Here's how the part is built. I have some questions about the finished solid (model axes, mm). A direction names the side the tool comes from. Coordinates: 2 decimals unless noted, no trailing zeros. Loops run counter-clockwise (first coordinate to the right, second up) from the corner with the lowest first, then second, coordinate; pieces in that order, holes last. Notation, with made-up numbers: M 59,63.25 L 106,63.25 A26 cw 106,89.25 Z; hole C 0.5,63 d4. An arc over 180 degrees is marked long. Use one line per item in the form item = value. Start each with the question number.
(1) Thinking about a two-plate mould opening in Z: for faces 1 (the cylindrical face through (81.769, 10.14, 82.675)), 2 (the flat face through (11.7, 9.86, 97.58)), 3 (the flat face through (-44.38, 10, -1)), 4 (the flat face through (29.375, 10, 0)), which applies, +Z half, -Z half, draft (parallel to the pull), parting line (faces both ways), or undercut?
(2) Please list where these lines run through material, in increasing order: L1, parallel to Z at x = -7, y = 16; L2, parallel to Z at x = 7.5, y = 2; L3, parallel to X at y = 10, z = -14.
(3) Imagine slicing it at D-D, the plane x = 48. Please give me the cut outline in (y, z).
(4) Will these pins go through, and if not, where does the flat tip stop? P1, Ø3, axis at x = 117.5, y = 4, coming from the -Z side; P2, Ø1.5, axis at y = 11.5, z = 75, coming from the +X side; P3, Ø8, axis at x = 60, y = 4.5, coming from the -Z side; P4, Ø5, axis at x = 83.76, z = 84.5, coming from the +Y side.
(5) Imagine slicing it at B-B, the plane x = -26.5. Please give me the cut outline in (y, z), and give its area (3 significant figures).
(6) Imagine slicing it at A-A, the plane z = 24.5. Please give me the cut outline in (x, y), and give its area (3 significant figures).
(7) Imagine slicing it at C-C, the plane y = 6.75. Please give me the cut outline in (x, z).
(8) On a 3-axis mill with a long thin cutter (end or side, diameter ignored), from which of +Z, -Z, +X, -X, +Y, -Y can I reach the whole of each face in a straight line? I mean faces 5 (the flat face through (1, 10, -43.108)), 6 (the flat face through (-29.375, 10, 0)). Say none if no direction works.
```python
from build123d import *

# Parameters (mm, degrees)
SKETCH1_W           = 58.749440694
SKETCH1_H           = 53.662909032
BOSS_EXTRUDE1_DEPTH = 20
SKETCH2_R           = 2.7
CUT_EXTRUDE1_DEPTH  = 20
SKETCH4_R           = 3


with BuildPart() as part:
    # Sketch1 → Boss-Extrude1 (new body)
    with BuildSketch(Plane(origin=(0, 0, 0), x_dir=(1, 0, 0), z_dir=(0, 1, 0))):
        Polygon((69.363086635, -153.592317311), (152.403813045, -68.102011951), (44.37998875, 43.108355834), (-44.37998875, 43.108355834), (-44.37998875, -43.108355834), align=None)
        Rectangle(SKETCH1_W, SKETCH1_H, mode=Mode.SUBTRACT)
    extrude(amount=BOSS_EXTRUDE1_DEPTH)

    # Sketch2 → Cut-Extrude1 (cut)
    with BuildSketch(Plane(origin=(0, 20, 0), x_dir=(1, 0, 0), z_dir=(0, 1, 0))):
        with Locations((83.759038646, -84.499957196)):
            Circle(SKETCH2_R)
    extrude(amount=-CUT_EXTRUDE1_DEPTH, mode=Mode.SUBTRACT)

    # Cut-Sweep1: sweep along a path in Sketch3
    with BuildLine(Plane.XZ) as cut_sweep1_path:
        CenterArc((83.759038646, 84.499957196), 15, 0, 360)
    # Sketch4 → Cut-Sweep1 (sweep, cut)
    with BuildSketch(Plane(origin=(0, 0, 0), x_dir=(0.703986253, 0, 0.710213599), z_dir=(-0.710213599, 0, 0.703986253))):
        with Locations((103.97823045, 0)):
            Circle(SKETCH4_R)
    sweep(path=cut_sweep1_path.line, mode=Mode.SUBTRACT)


solid = part.part
```
Answer:
q1.face_1 = undercut
q1.face_2 = +Z half
q1.face_3 = draft
q1.face_4 = undercut
q2.L1 = -43.11 to -26.83, 26.83 to 79.42
q2.L2 = -43.11 to -26.83, 26.83 to 93.5
q2.L3 = -44.38 to -29.37, 29.37 to 72.65
q3.outline = M 0,-39.38 L 20,-39.38 L 20,132.84 L 0,132.84 Z
q4.P1 = 30.62
q4.P2 = 146.43
q4.P3 = -31.15
q4.P4 = through
q5.outline = M 0,-43.11 L 20,-43.11 L 20,-26.83 L 0,-26.83 Z; M 0,26.83 L 20,26.83 L 20,60.48 L 0,60.48 Z
q5.area = 998 mm²
q6.outline = M -44.38,0 L -29.37,0 L -29.37,20 L -44.38,20 Z; M 29.37,0 L 110.05,0 L 110.05,20 L 29.37,20 Z
q6.area = 1,910 mm²
q7.outline = M -44.38,-43.11 L 44.38,-43.11 L 152.4,68.1 L 69.36,153.59 L -44.38,43.11 Z; hole M -29.37,-26.83 L 29.37,-26.83 L 29.37,26.83 L -29.37,26.83 Z; hole C 83.76,84.5 d5.4
q8.face_5 = -Z, +X, -X, +Y, -Y
q8.face_6 = +Y, -Y
